Could you check a few things on this model? Use its own coordinates, in mm. Face numbers are marked on the shaded views. Give positions to 0.01 mm unless a question says otherwise; leave off trailing zeros. Loops run counter-clockwise (first coordinate to the right, second up) from the corner with the lowest first, then second, coordinate; pieces in that order, holes last. Notation, with made-up numbers: M 45,23.5 L 100,23.5 A11 ccw 100,42.5 Z; hole C -22,-20.5 d1. An arc over 180 degrees is marked long. Use CSV: the item, a comma, the result in double quotes.
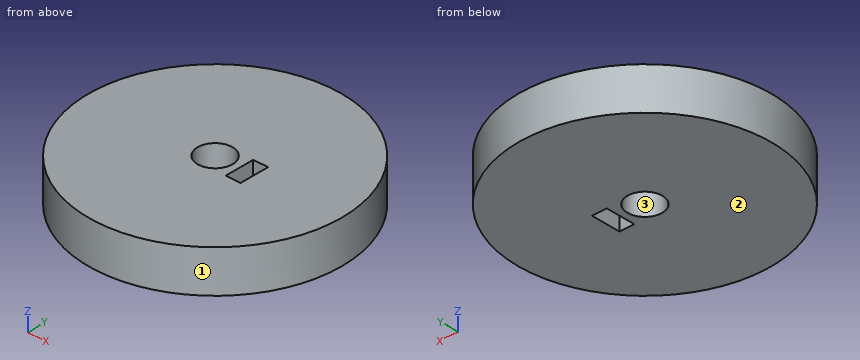
```python
from build123d import *

# Parameters (mm, degrees)
SKETCH1_R           = 45
SKETCH1_R_2         = 6.2
SKETCH1_W           = 5.3
SKETCH1_H           = 10.6
BOSS_EXTRUDE1_DEPTH = 15


with BuildPart() as part:
    # Sketch1 → Boss-Extrude1 (new body)
    with BuildSketch(Plane.XY):
        with Locations((-85.316632571, -12.372200494)):
            Circle(SKETCH1_R)
        with Locations((-85.316632571, -12.372200494)):
            Circle(SKETCH1_R_2, mode=Mode.SUBTRACT)
        with Locations((-73.984503587, -12.372200494)):
            Rectangle(SKETCH1_W, SKETCH1_H, mode=Mode.SUBTRACT)
    extrude(amount=BOSS_EXTRUDE1_DEPTH)


solid = part.part
```
1. I want a section at D-D, the plane x = -55. List the corners of the cut face in (y, z) for me, then the cut area to 3 significant figures.
Outcome:
outline,"M -45.63,0 L 20.88,0 L 20.88,15 L -45.63,15 Z"
area,"998 mm2"
2. If we mould it in two halves opening along X, with no side actions, what happens to the marked faces 1, 2 and 3? For each: +X half, -X half, draft (parallel to the pull), parting line (faces both ways), or undercut.
Outcome:
face 1,"parting line"
face 2,"draft"
face 3,"undercut"
3. I'm going to push flat-ended pins straight in: pin 1 Ø3 at (x, z) = (-71.5, 2.5) entering from +Y; pin 2 Ø2 at (x, z) = (-50, 12.5) entering from +Y; pin 3 Ø6 at (x, z) = (-74.5, 10.5) entering from +Y. Where does each tip first touch, or does it pass through?
Outcome:
pin 1,"y = 30.91"
pin 2,"y = 16.74"
pin 3,"y = 31.94"
4. I want a section at C-C, the plane y = -47. List the corners of the cut face in (x, z) for me.
Outcome:
outline,"M -114.06,0 L -56.58,0 L -56.58,15 L -114.06,15 Z"
5. I want a section at A-A, the plane x = -85.5. List the corners of the cut face in (y, z) for me.
Outcome:
outline,"M -57.37,0 L -18.57,0 L -18.57,15 L -57.37,15 Z; M -6.17,0 L 32.63,0 L 32.63,15 L -6.17,15 Z"
6. I want a section at B-B, the plane z = 11.25. List the corners of the cut face in (x, y) for me.
Outcome:
outline,"C -85.32,-12.37 d90; hole C -85.32,-12.37 d12.4; hole M -76.63,-17.67 L -71.33,-17.67 L -71.33,-7.07 L -76.63,-7.07 Z"
7. Please list where these lines run through material, in increasing order: line 1 (X direction, y = -9, z = 6); line 2 (X direction, y = -16.5, z = 13); line 3 (X direction, y = 22, z = 12).
Outcome:
line 1,"-130.19 to -90.52, -80.11 to -76.63, -71.33 to -40.44"
line 2,"-130.13 to -89.94, -80.69 to -76.63, -71.33 to -40.51"
line 3,"-114.36 to -56.27"
